Verification items for the finished model (mm, model axes). A direction names the side the tool comes from. Round coordinates to 2 decimals unless told otherwise and drop trailing zeros. Order: outer loops, then holes, each group sorted by start corner. A loop starts at its lowest first (then second) coordinate and runs counter-clockwise, first axis right, second up. Notation, with made-up numbers: M 19,53.25 L 31,53.25 A27 cw 31,86.25 Z; hole C 63,-9.5 d7. An arc over 180 degrees is marked long. Use one line per item in the form item = value. Start each with the question number.
Item 1: Go/stop test with flat-tipped pins: pin 1 Ø2.5 at (y, z) = (0, -3.5) entering from -X; pin 2 Ø1 at (x, y) = (-9.5, 2) entering from -Z; pin 3 Ø4 at (x, y) = (-46, 0) entering from -Z. Record where each tip stops, or that it passes through.
Item 2: Tool access check on faces 4 (the flat face through (-40, 0, 3)), 5 (the cylindrical face through (-15, -3, 0)), 6 (the cylindrical face through (-34.06, -1.08, 4.88)), 7 (the flat face through (0, 0, 0)), 8 (the flat face through (-40, 0, -3)). Record the directions out of +Z, -Z, +X, -X, +Y, -Y that give a thin tool (end or side, any length) a straight path to the whole face; none if there is none.
Item 3: Cross-section at B-B on x = -46. Enter the section's corners in (y, z), then the cut area to 3 significant figures.
Item 4: Cross-section at D-D on x = -3.5. Enter the section's corners in (y, z).
Item 5: Release check for a two-part mould opening along Y. For faces 1 (the flat face through (-29, -1, 3)), 2 (the cylindrical face through (-42.912, 4.477, -0.457)), 3 (the cylindrical face through (-47.464, -0.325, -0.021)) record: +Y half, -Y half, draft (parallel to the pull), parting line (faces both ways), or undercut.
Item 6: Thickness scan on probe 1 along X at (y, z) = (0, 0.5); probe 2 along X at (y, z) = (1.25, 2); probe 3 along Z at (x, y) = (-13, -0.25). Record the ranges inside material, lowest first. Write a range as [from, to].
from build123d import *

# Parameters (mm, degrees)
FILLET_1_R          = 2
SKETCH_2_R          = 7.321356554
SKETCH_2_W          = 3
SKETCH_2_H          = 11.961651185
CUT_EXTRUDE_1_DEPTH = 11
SKETCH_3_R          = 1.5
CUT_EXTRUDE_2_DEPTH = 3
FILLET_2_R          = 0.5


with BuildPart() as part:
    # 草图1 → 旋转1 (revolve)
    with BuildSketch(Plane.XY):
        Polygon((0, 0), (0, 3), (-29, 3), (-29, 5), (-39, 5), (-39, 4.5), (-51, 4.5), (-51, 0), align=None)
    revolve(axis=Axis((0, 0, 0), (-1, 0, 0)))

    # 圆角1
    fillet_1_edges = [part.edges().sort_by_distance(p)[0] for p in [
        (-51, -4.5, 0),
    ]]
    fillet(fillet_1_edges, radius=FILLET_1_R)

    # 草图2 → 切除-拉伸1 (cut)
    with BuildSketch(Plane.ZY.offset(51)):
        Circle(SKETCH_2_R)
        with Locations((0, -0.178000761)):
            Rectangle(SKETCH_2_W, SKETCH_2_H, mode=Mode.SUBTRACT)
    extrude(amount=-CUT_EXTRUDE_1_DEPTH, mode=Mode.SUBTRACT)

    # 草图3 → 切除-拉伸2 (cut)
    with BuildSketch(Plane(origin=(0, 0, -1.5), x_dir=(-1, 0, 0), z_dir=(0, 0, -1))):
        with Locations(Location((46, 0, 0), (0, 0, 90))):
            Circle(SKETCH_3_R)
    extrude(amount=-CUT_EXTRUDE_2_DEPTH, mode=Mode.SUBTRACT)

    # 圆角2
    fillet_2_edges = [part.edges().sort_by_distance(p)[0] for p in [
        (-39, -5, 0),
        (-29, -5, 0),
        (0, -3, 0),
    ]]
    fillet(fillet_2_edges, radius=FILLET_2_R - 0.0001)  # a hair under: the kernel refuses the full size


solid = part.part
Output values:
q1.pin_1 = -40
q1.pin_2 = -2.6
q1.pin_3 = -1.5
q2.face_4 = +Z, -X, +Y, -Y
q2.face_5 = +X
q2.face_6 = +X, -X
q2.face_7 = +Z, -Z, +X, +Y, -Y
q2.face_8 = -Z, -X, +Y, -Y
q3.outline = M -4.24,-1.5 L -1.5,-1.5 L -1.5,1.5 L -4.24,1.5 A4.5 ccw Z; M 1.5,-1.5 L 4.24,-1.5 A4.5 ccw 4.24,1.5 L 1.5,1.5 Z
q3.area = 17.5 mm2
q4.outline = C 0,0 d6
q5.face_1 = draft
q5.face_2 = parting line
q5.face_3 = undercut
q6.probe_1 = [-51, -47.5], [-44.5, 0]
q6.probe_2 = [-40, 0]
q6.probe_3 = [-2.99, 2.99]
